Could you check a few things on this drawing? It's one solid part, dimensions in mm from its lowest x, y, z. Give positions to 0.01 mm unless a question says otherwise; leave off trailing zeros. Loops run counter-clockwise (first coordinate to the right, second up) from the corner with the lowest first, then second, coordinate; pieces in that order, holes last. Notation, with made-up numbers: M 53.5,67.5 L 62.5,67.5 A28 ccw 62.5,94.5 Z; hole C 30.25,54 d5. An arc over 180 degrees is marked long. Answer as a JSON object with one key per item and string values.
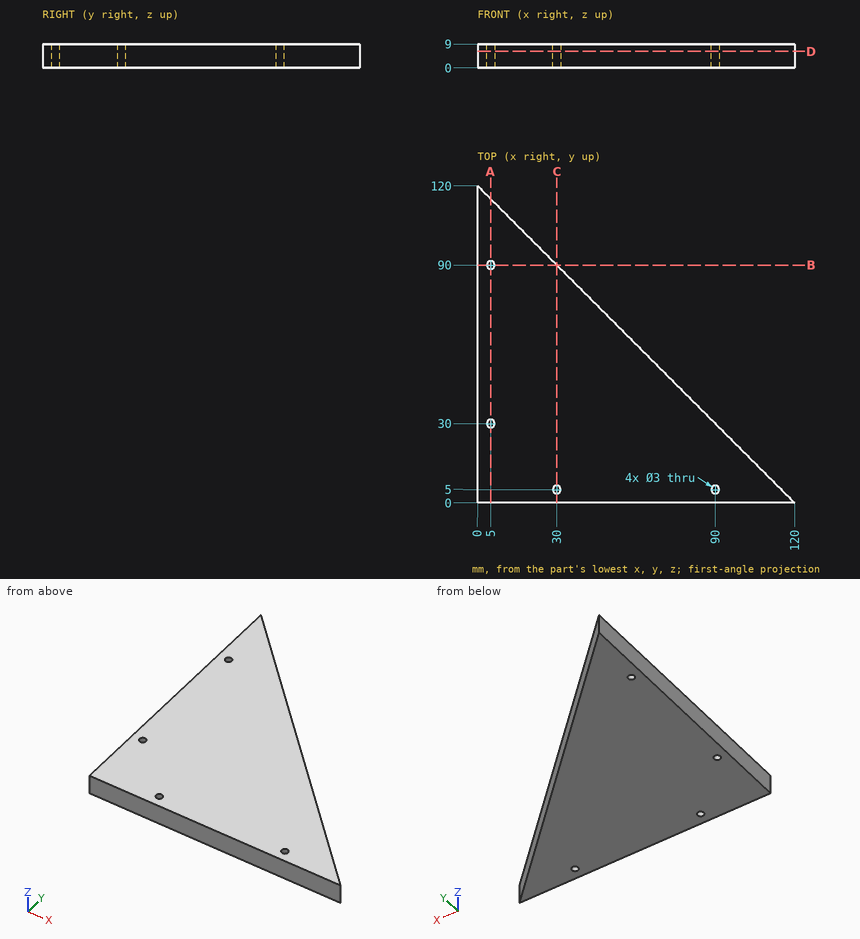
1) Suppose I cut it at A-A, the plane x = 5. Write out the boundary of the cut face in (y, z), and give its area (3 significant figures).
Answer list:
{"outline": "M 0,0 L 28.5,0 L 28.5,9 L 0,9 Z; M 31.5,0 L 88.5,0 L 88.5,9 L 31.5,9 Z; M 91.5,0 L 115,0 L 115,9 L 91.5,9 Z", "area": "981 mm^2"}
2) Suppose I cut it at B-B, the plane y = 90. Write out the boundary of the cut face in (x, z), and give its area (3 significant figures).
Answer list:
{"outline": "M 0,0 L 3.5,0 L 3.5,9 L 0,9 Z; M 6.5,0 L 30,0 L 30,9 L 6.5,9 Z", "area": "243 mm^2"}
3) Will these pins go through, and if not, where does the flat tip stop? pin 1 Ø5 at (x, z) = (43, 7) entering from +Y; pin 2 Ø4 at (y, z) = (60, 3) entering from +X.
Answer list:
{"pin 1": "y = 79.5", "pin 2": "x = 62"}
4) Suppose I cut it at D-D, the plane z = 6.25. Write out the boundary of the cut face in (x, y), and give its area (3 significant figures).
Answer list:
{"outline": "M 0,0 L 120,0 L 0,120 Z; hole C 5,30 d3; hole C 5,90 d3; hole C 30,5 d3; hole C 90,5 d3", "area": "7,170 mm^2"}
5) Suppose I cut it at C-C, the plane x = 30. Write out the boundary of the cut face in (y, z), and give its area (3 significant figures).
Answer list:
{"outline": "M 0,0 L 3.5,0 L 3.5,9 L 0,9 Z; M 6.5,0 L 90,0 L 90,9 L 6.5,9 Z", "area": "783 mm^2"}
6) Please list where these lines run through material, in increasing order: line 1 along Y through (x, z) = (90, 5.75); line 2 along Y through (x, z) = (5, 5.75); line 3 along X through (y, z) = (26.5, 5.25). Write a range as from..to.
Answer list:
{"line 1": "0..3.5, 6.5..30", "line 2": "0..28.5, 31.5..88.5, 91.5..115", "line 3": "0..93.5"}
